Geometry: final body of the model. Coordinates: model frame, mm. Face numbers are marked on the shaded views. A direction names the side the tool comes from. Round coordinates to 2 decimals unless told otherwise and drop trailing zeros. Order: outer loops, then holes, each group sorted by start corner. A loop starts at its lowest first (then second) coordinate and runs counter-clockwise, first axis right, second up. Notation, with made-up numbers: (-30.75, 72) -> (14.25, 72) arc R27 ccw to (14.25, 92) -> close; hole circle Ø9 at (39.25, 89.5). An arc over 180 degrees is marked (long way). Put each result on its own line as item: value.
```python
from build123d import *

# Parameters (mm, degrees)
SKETCH1_R           = 17
BOSS_EXTRUDE1_DEPTH = 25
BOSS_EXTRUDE5_START = 8
SKETCH1_6_R         = 19
SKETCH1_6_R_2       = 17
BOSS_EXTRUDE5_DEPTH = 8
BOSS_EXTRUDE6_DEPTH = 15
SKETCH4_R           = 16
BOSS_EXTRUDE7_DEPTH = 15
BOSS_EXTRUDE8_START = 5
SKETCH5_R           = 17
BOSS_EXTRUDE8_DEPTH = 5


with BuildPart() as part:
    # Sketch1 → Boss-Extrude1 (new body)
    with BuildSketch(Plane(origin=(0, 0, 0), x_dir=(0, 0, -1), z_dir=(1, 0, 0))):
        Circle(SKETCH1_R)
    extrude(amount=-BOSS_EXTRUDE1_DEPTH)

    # Sketch1_6 → Boss-Extrude5 (add)
    # profile 1 of 2: a face of its own
    with BuildSketch(Plane(origin=(0, 0, 0), x_dir=(0, 0, -1), z_dir=(1, 0, 0)).offset(BOSS_EXTRUDE5_START)):
        Circle(SKETCH1_6_R)
        Circle(SKETCH1_6_R_2, mode=Mode.SUBTRACT)
    # profile 2 of 2: a face of its own
    with BuildSketch(Plane(origin=(0, 0, 0), x_dir=(0, 0, -1), z_dir=(1, 0, 0)).offset(BOSS_EXTRUDE5_START)):
        Circle(SKETCH1_6_R_2)
    extrude(amount=-BOSS_EXTRUDE5_DEPTH)

    # Sketch2 → Boss-Extrude6 (add)
    with BuildSketch(Plane(origin=(8, 0, 0), x_dir=(0, 0, -1), z_dir=(1, 0, 0))):
        with BuildLine():
            ThreePointArc((-13.668094758, 40.943123461), (0, 46), (13.668094758, 40.943123461))
            ThreePointArc((13.668094758, 40.943123461), (33.683444249, 16.469257624), (44, -13.416407865))
            ThreePointArc((44, -13.416407865), (0, -46), (-44, -13.416407865))
            ThreePointArc((-44, -13.416407865), (-33.683444249, 16.469257624), (-13.668094758, 40.943123461))
        make_face()
    boss_extrude6 = extrude(amount=BOSS_EXTRUDE6_DEPTH)

    # Sketch4 → Boss-Extrude7 (add)
    with BuildSketch(Plane(origin=(23, 0, 0), x_dir=(0, 0, -1), z_dir=(1, 0, 0))):
        with Locations((0, 25)):
            Circle(SKETCH4_R)
    boss_extrude7 = extrude(amount=BOSS_EXTRUDE7_DEPTH)

    # Mirror1: Boss-Extrude6, Boss-Extrude7 across plane
    add(boss_extrude6.mirror(Plane(origin=(38, 25, 0), x_dir=(0, 0, 1), z_dir=(1, 0, 0))))
    add(boss_extrude7.mirror(Plane(origin=(38, 25, 0), x_dir=(0, 0, 1), z_dir=(1, 0, 0))))

    # Sketch5 → Boss-Extrude8 (add)
    with BuildSketch(Plane(origin=(68, 0, 0), x_dir=(0, 0, -1), z_dir=(1, 0, 0)).offset(BOSS_EXTRUDE8_START)):
        Circle(SKETCH5_R)
    extrude(amount=-BOSS_EXTRUDE8_DEPTH)


solid = part.part
```
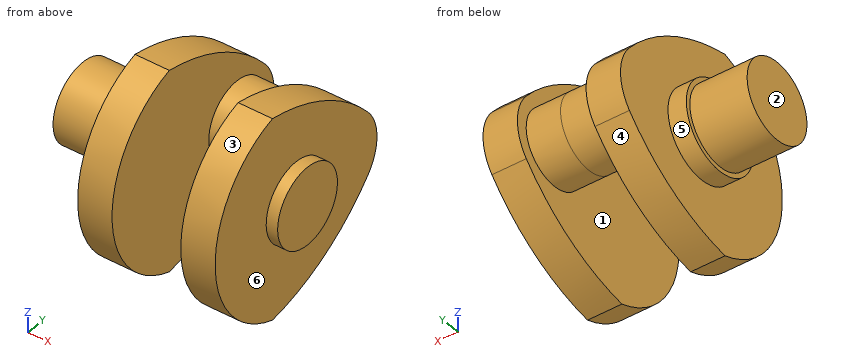
1. Contact query for flat-ended pins moving along their axis: P1, Ø10, axis at y = -21.5, z = 32, coming from the -X side; P2, Ø4, axis at x = 5, y = 3.5, coming from the -Z side; P3, Ø1, axis at x = 39, y = 25.5, coming from the -Z side. Output: stop coordinate, or through.
Ans:
P1: x = 8
P2: z = -18.94
P3: z = -16
2. Cut plane B-B on z = -31. Return loops of the section in (x, y).
Ans:
outline: (8, -33.99) -> (23, -33.99) -> (23, 20.97) -> (8, 20.97) -> close; (53, -33.99) -> (68, -33.99) -> (68, 20.97) -> (53, 20.97) -> close
3. Set-up query: the marked faces 4, 5 and 6. Return all of +Z, -Z, +X, -X, +Y, -Y with unobstructed straight access to the full face (end or side cutting, diameter ignored); none if empty.
Ans:
face 4: -Z, +X, -X, +Y
face 5: -X
face 6: +X
4. Cut plane C-C on z = 0. Return loops of the section in (x, y), and give its area (3 significant figures).
Ans:
outline: (-25, -17) -> (0, -17) -> (0, -19) -> (8, -19) -> (8, -46) -> (23, -46) -> (23, 9) -> (53, 9) -> (53, -46) -> (68, -46) -> (68, -17) -> (73, -17) -> (73, 17) -> (68, 17) -> (68, 46) -> (53, 46) -> (53, 41) -> (23, 41) -> (23, 46) -> (8, 46) -> (8, 19) -> (0, 19) -> (0, 17) -> (-25, 17) -> close
area: 5,040 mm²
5. Draft query along X for the marked faces 1, 2 and 3. Return one class per face: +X half, -X half, draft (parallel to the pull), parting line (faces both ways), or undercut.
Ans:
face 1: undercut
face 2: -X half
face 3: draft
6. Material intervals for probe 1 along X at (y, z) = (20, 31.5); probe 2 along X at (y, z) = (30.5, 7.5); probe 3 along Z at (x, y) = (2.5, 1), sorted ascending.
Ans:
probe 1: 8 to 23, 53 to 68
probe 2: 8 to 68
probe 3: -18.97 to 18.97
7. Cut plane A-A on y = -26. Return loops of the section in (x, z).
Ans:
outline: (8, -37.95) -> (23, -37.95) -> (23, 37.95) -> (8, 37.95) -> close; (53, -37.95) -> (68, -37.95) -> (68, 37.95) -> (53, 37.95) -> close
8. Cut plane D-D on y = 25. Return loops of the section in (x, z), and give its area (3 significant figures).
Ans:
outline: (8, -28.27) -> (23, -28.27) -> (23, -16) -> (53, -16) -> (53, -28.27) -> (68, -28.27) -> (68, 28.27) -> (53, 28.27) -> (53, 16) -> (23, 16) -> (23, 28.27) -> (8, 28.27) -> close
area: 2,660 mm²
